Here's the drawing with two shaded views (mm, measured from the low corner). I have some questions. A direction names the side the tool comes from. Give positions to 0.01 mm unless a question says otherwise; leave off trailing zeros. Loops run counter-clockwise (first coordinate to the right, second up) from the corner with the lowest first, then second, coordinate; pieces in that order, holes last. Notation, with made-up numbers: (-33, 77.25) - (-20, 77.25) arc R37 ccw to (-20, 116.25) - close; hole circle Ø3 at (1.25, -38.75). An arc over 180 degrees is marked (long way). Use one line per item in the form item = value.
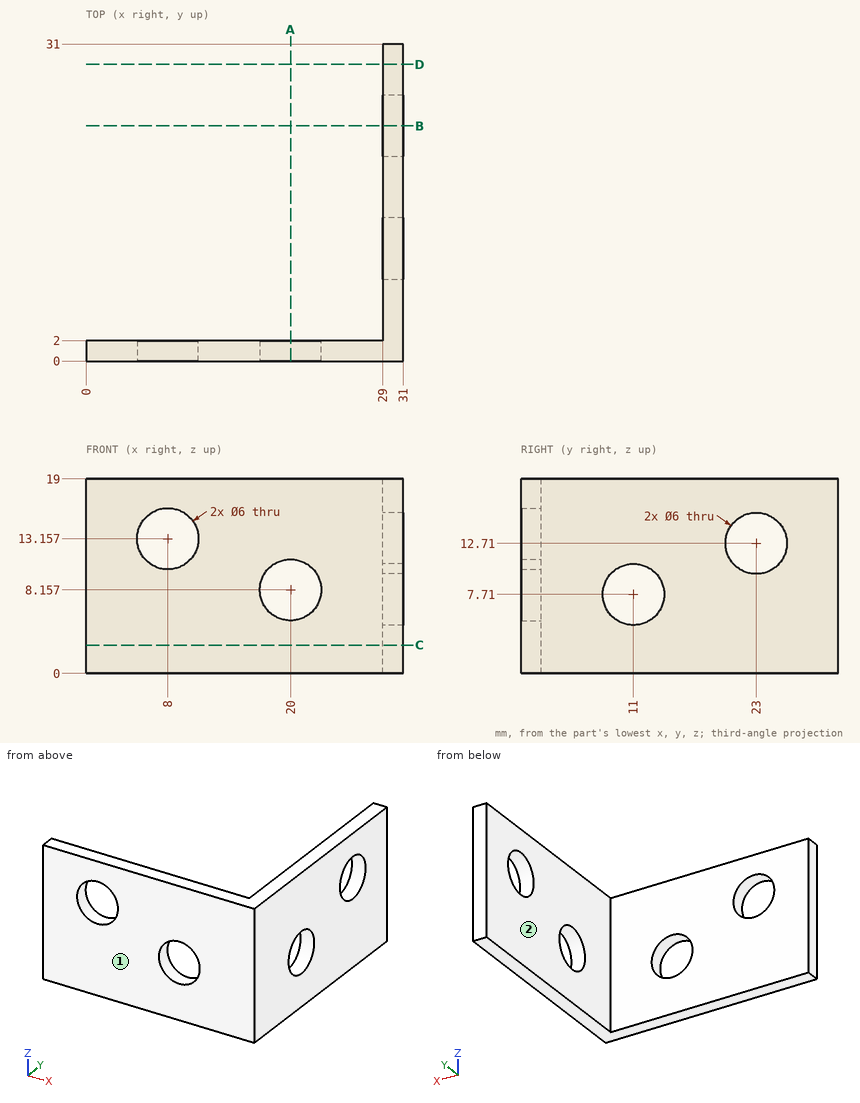
(1) If we section it at A-A (x = 20): List the corners of the cut face in (y, z) for me.
Geometry says:
outline = (0, 0) - (2, 0) - (2, 5.16) - (0, 5.16) - close; (0, 11.16) - (2, 11.16) - (2, 19) - (0, 19) - close
(2) If I drill on probe 1 along Z at (x, y) = (20, 1.65); probe 2 along Z at (x, y) = (29.55, 23); probe 3 along X at (y, z) = (15, 7), over which ranges is the centre line in solid material (lowest first)?
Geometry says:
probe_1 = 0 to 5.16, 11.16 to 19
probe_2 = 0 to 9.71, 15.71 to 19
probe_3 = 29 to 31
(3) For P1, Ø10, axis at x = 5, z = 4, coming from the +Y side; P2, Ø3, axis at x = 16.5, y = 4.5, coming from the -Z side (3 decimals), each with a flat end and sliding along its axis, tell me the tip position at first contact or that it passes through.
Geometry says:
P1 = 2
P2 = through
(4) For the marked faces 1 and 2, which set-ups out of +Z, -Z, +X, -X, +Y, -Y let a thin tool reach every point of the face, with its end or its side?
Geometry says:
face_1 = +Z, -Z, +X, -X, -Y
face_2 = +Z, -Z, -X, +Y
(5) If we section it at D-D (y = 29): List the corners of the cut face in (x, z) for me, plus the area to 3 significant figures.
Geometry says:
outline = (29, 0) - (31, 0) - (31, 19) - (29, 19) - close
area = 38.0 mm²
(6) If we section it at C-C (z = 2.75): List the corners of the cut face in (x, y) for me.
Geometry says:
outline = (0, 0) - (31, 0) - (31, 31) - (29, 31) - (29, 2) - (0, 2) - close
(7) If we section it at B-B (y = 23): List the corners of the cut face in (x, z) for me, plus the area to 3 significant figures.
Geometry says:
outline = (29, 0) - (31, 0) - (31, 9.71) - (29, 9.71) - close; (29, 15.71) - (31, 15.71) - (31, 19) - (29, 19) - close
area = 26.0 mm²
